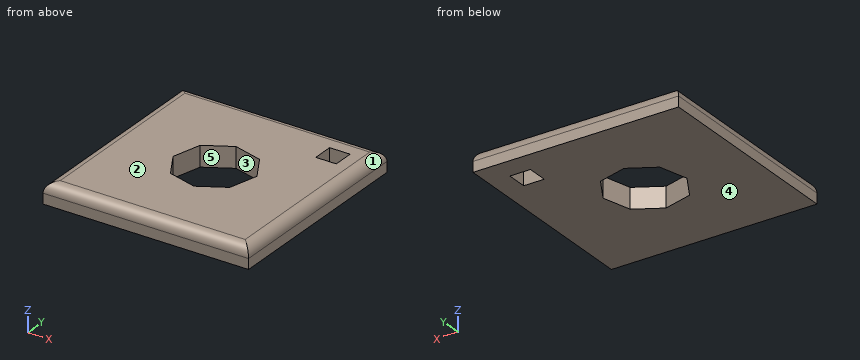
from build123d import *

# Parameters (mm, degrees)
F0_W     = 100
F0_H     = 100
F2_DEPTH = 10
F3_R     = 5
F4_DEPTH = 106.8
F5_W     = 10
F5_H     = 10
F6_DEPTH = 90.6


with BuildPart() as f2:
    # F0 (on Top) → F2 (new body)
    with BuildSketch(Plane.XY):
        Rectangle(F0_W, F0_H)
    extrude(amount=F2_DEPTH)

    # F3
    f3_edges = [f2.edges().sort_by_distance(p)[0] for p in [
        (50, 0, 10),
        (0, 50, 10),
        (-50, 0, 10),
        (0, -50, 10),
    ]]
    fillet(f3_edges, radius=F3_R)

    # F1 (on face) → F4 (cut)
    with BuildSketch(Plane.XY):
        Polygon((18.788767, 2.403422), (11.586189, 14.98514), (-2.403422, 18.788767), (-14.98514, 11.586189), (-18.788767, -2.403422), (-11.586189, -14.98514), (2.403422, -18.788767), (14.98514, -11.586189), align=None)
    extrude(amount=F4_DEPTH, mode=Mode.SUBTRACT)

    # F5 (on face) → F6 (cut)
    with BuildSketch(Plane.XY.offset(10)):
        with Locations((34.426235, 34.082789)):
            Rectangle(F5_W, F5_H)
    extrude(amount=-F6_DEPTH, mode=Mode.SUBTRACT)


solid = f2.part
Model file for the job. Use its own axes, mm. Face numbers are marked on the shaded views. A direction names the side the tool comes from. Give positions to 0.01 mm unless a question says otherwise; leave off trailing zeros. Loops run counter-clockwise (first coordinate to the right, second up) from the corner with the lowest first, then second, coordinate; pieces in that order, holes last.
1) Wall check: line 1 (Z direction, x = 23, y = 45.5); line 2 (Y direction, x = 10.5, z = 5.75); line 3 (Y direction, x = -14.5, z = 4). Give the ranges that are in metal, low to high.
2) Saw through at A-A (y = 37.5). Write the cut outline in (x, z).
3) Saw through at D-D (z = 8.5). Write the cut outline in (x, y).
4) Tool access for the marked faces 4 and 5: list every direction of +Z, -Z, +X, -X, +Y, -Y with a clear straight run to the whole face (end or side of a thin tool).
5) Saw through at B-B (x = 31.5). Write the cut outline in (y, z), plus the area to 3 significant figures.
6) Flat gauge pin, fed straight in: pin 1 Ø1.5 at (y, z) = (14.5, 6) entering from +X. Where does the tip first touch, or does it go through?
7) Saw through at C-C (z = 3.25). Write the cut outline in (x, y).
8) Pull direction X, two halves, no side cores. Call the marked faces 1, 2 and 3: +X half, -X half, draft (parallel to the pull), parting line (faces both ways), or undercut.
Answer block:
1. line 1: z = 0 to 9.97
1. line 2: y = -49.94 to -14.15, 15.28 to 49.94
1. line 3: y = -50 to -9.9, 11.86 to 50
2. outline: (-50, 0) - (29.43, 0) - (29.43, 10) - (-45, 10) arc R5 ccw to (-50, 5) - close; (39.43, 0) - (50, 0) - (50, 5) arc R5 ccw to (45, 10) - (39.43, 10) - close
3. outline: (-48.57, -48.57) - (48.57, -48.57) - (48.57, 48.57) - (-48.57, 48.57) - close; hole (-18.79, -2.4) - (-11.59, -14.99) - (2.4, -18.79) - (14.99, -11.59) - (18.79, 2.4) - (11.59, 14.99) - (-2.4, 18.79) - (-14.99, 11.59) - close; hole (29.43, 29.08) - (39.43, 29.08) - (39.43, 39.08) - (29.43, 39.08) - close
4. face 4: -Z, +X, -X, +Y, -Y
4. face 5: +Z, -Z
5. outline: (-50, 0) - (29.08, 0) - (29.08, 10) - (-45, 10) arc R5 ccw to (-50, 5) - close; (39.08, 0) - (50, 0) - (50, 5) arc R5 ccw to (45, 10) - (39.08, 10) - close
5. area: 889 mm2
6. pin 1: stops at x = 49.99
7. outline: (-50, -50) - (50, -50) - (50, 50) - (-50, 50) - close; hole (-18.79, -2.4) - (-11.59, -14.99) - (2.4, -18.79) - (14.99, -11.59) - (18.79, 2.4) - (11.59, 14.99) - (-2.4, 18.79) - (-14.99, 11.59) - close; hole (29.43, 29.08) - (39.43, 29.08) - (39.43, 39.08) - (29.43, 39.08) - close
8. face 1: +X half
8. face 2: draft
8. face 3: undercut
